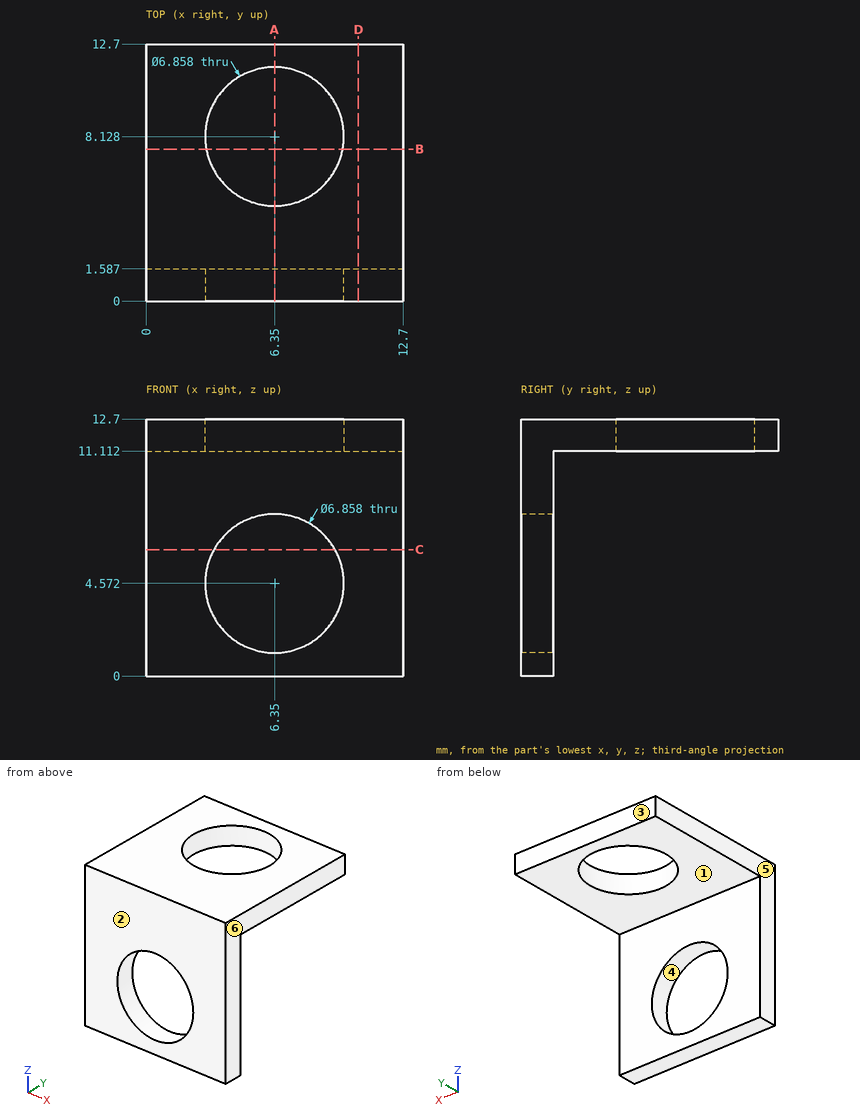
Design review of the part shown in the three views and the two pictorial views. Dimensions are in mm from the part's minimum x, y and z. A direction names the side the tool comes from. Round coordinates to 2 decimals unless told otherwise and drop trailing zeros. Loops run counter-clockwise (first coordinate to the right, second up) from the corner with the lowest first, then second, coordinate; pieces in that order, holes last. Notation, with made-up numbers: M 4,47 L 54,47 A16 ccw 54,52 Z; hole C 87.25,-27 d9. An arc over 180 degrees is marked long. Put each result on its own line as item: value.
Q1. Consider section D-D, the plane x = 10.5. Give the boundary of the cut face in (y, z).
Result set:
outline: M 0,0 L 1.59,0 L 1.59,11.11 L 12.7,11.11 L 12.7,12.7 L 0,12.7 Z
Q2. Consider section A-A, the plane x = 6.35. Give the boundary of the cut face in (y, z).
Result set:
outline: M 0,0 L 1.59,0 L 1.59,1.14 L 0,1.14 Z; M 0,8 L 1.59,8 L 1.59,11.11 L 4.7,11.11 L 4.7,12.7 L 0,12.7 Z; M 11.56,11.11 L 12.7,11.11 L 12.7,12.7 L 11.56,12.7 Z
Q3. Consider section B-B, the plane y = 7.5. Give the boundary of the cut face in (x, z).
Result set:
outline: M 0,11.11 L 2.98,11.11 L 2.98,12.7 L 0,12.7 Z; M 9.72,11.11 L 12.7,11.11 L 12.7,12.7 L 9.72,12.7 Z
Q4. Mouldability with a two-part tool opening along X and no side actions: class the marked faces 3, 4, 5 and 6 as released by +X, released by -X, zero draft, split by the parting line, or undercut.
Result set:
face 3: zero draft
face 4: undercut
face 5: released by -X
face 6: released by +X
Q5. To check wall thickness, follow L1, parallel to Y at x = 6.35, z = 12.4; L2, parallel to Z at x = 6.35, y = 1; L3, parallel to X at y = 8, z = 12.25. State the ranges of each line that lie inside material, in increasing order.
Result set:
L1: y = 0 to 4.7, 11.56 to 12.7
L2: z = 0 to 1.14, 8 to 12.7
L3: x = 0 to 2.92, 9.78 to 12.7
Q6. Machinability: for the marked faces 1 and 2, which of the approach directions +Z, -Z, +X, -X, +Y, -Y give a long, thin tool a straight path to every point of the face, cutting with its end or side? Answer none if there is none.
Result set:
face 1: -Z, +X, -X, +Y
face 2: +Z, -Z, +X, -X, -Y
Q7. Consider section C-C, the plane z = 6.25. Give the boundary of the cut face in (x, y).
Result set:
outline: M 0,0 L 3.36,0 L 3.36,1.59 L 0,1.59 Z; M 9.34,0 L 12.7,0 L 12.7,1.59 L 9.34,1.59 Z
